The listing builds one solid part. Answer for the finished solid, in the listing's coordinates (mm). A direction names the side the tool comes from. Round coordinates to 2 decimals unless told otherwise and drop trailing zeros. Loops run counter-clockwise (first coordinate to the right, second up) from the corner with the lowest first, then second, coordinate; pieces in that order, holes last. Notation, with made-up numbers: M -26,-21 L 27,-21 A9 cw 27,-7 Z; hole C 83.5,-31 d6. An arc over 180 degrees is marked long. Answer as a JSON object with one key per item and string values.
Solid Edge part; units mm, degrees
sketch "Sketch1" plane through (0, 0, 0) normal (0, 0, 1) x (1, 0, 0)
  line L0 (-49.9158, -24.6721) -> (49.9158, -24.6721)
  line L1 (49.9158, -24.6721) -> (49.9158, 24.6721)
  line L2 (49.9158, 24.6721) -> (-49.9158, 24.6721)
  line L3 (-49.9158, 24.6721) -> (-49.9158, -24.6721)
extrude "Protrusion1" add sketch "Sketch1" along normal blind 31.771
draft "Draft_1" angle 4 neutral plane through (0, 0, 0) normal (0, 0, 1) pull direction (0, 0, 1) face at (49.9158, -16.9415, 26.1581) face at (34.2755, 24.6721, 26.1581) face at (-49.9158, 16.9415, 26.1581) face at (-34.2755, -24.6721, 26.1581)
fillet "Round_1" radius 6 8 edges at (-48.8049, -23.5613, 15.8855) (0, -22.4505, 31.771) (-47.6941, 0, 31.771) (-48.8049, 23.5613, 15.8855) (0, 22.4505, 31.771) (47.6941, 0, 31.771) (48.8049, -23.5613, 15.8855) (48.8049, 23.5613, 15.8855)
sketch "Sketch2" plane through (0, 0, 31.771) normal (0, 0, 1) x (0, 1, 0)
  circle A0 centre (11.4247, -36.4932) radius 4
extrude "ExtrudedCutout_1" cut sketch "Sketch2" against normal blind 65.3593
sketch "Sketch3" plane through (20.8309, 11.4247, 31.771) normal (0, 0, 1) x (-1, 0, 0)
  circle A0 centre (0, 0) radius 4
  circle A1 centre (15.6623, 0) radius 4
  circle A2 centre (31.3245, 0) radius 4
extrude "ExtrudedCutout_2" cut sketch "Sketch3" against normal blind 66.2854
sketch "Sketch4" plane through (0, 0, 31.771) normal (0, 0, 1) x (0, 1, 0)
  line L0 (-6.6575, 36.4932) -> (-6.6575, 18.7397)
  line L1 (-6.6575, 18.7397) -> (-14.5479, 18.7397)
  line L2 (-14.5479, 18.7397) -> (-14.5479, 36.4932)
  line L3 (-14.5479, 36.4932) -> (-6.6575, 36.4932)
extrude "ExtrudedCutout_3" cut sketch "Sketch4" against normal blind 15.8022
shell "Thin_Wall_1" thickness 1 removed faces 1 at (-34.2755, -15.9546, 0)
Item 1: The part is cut by section D-D (x = 23). Give the vertices of the cut face in (y, z).
Values follow:
{"outline": "M -24.67,0 L -23.67,0 L -21.84,26.12 A5 cw -16.86,30.77 L 6.92,30.77 L 6.92,0 L 8.06,0 L 8.06,31.77 L -16.86,31.77 A6 ccw -22.84,26.19 Z; M 14.79,0 L 15.93,0 L 15.93,30.77 L 16.86,30.77 A5 cw 21.84,26.12 L 23.67,0 L 24.67,0 L 22.84,26.19 A6 ccw 16.86,31.77 L 14.79,31.77 Z"}
Item 2: Determine the mould class of faces 3 (the face through (-0.62, -23.77, 12.91)), 4 (the face through (34, 15, 0)), 5 (the face through (-27, -15.548, 23)) for opening direction Y: released by +Y, released by -Y, zero draft, split by the parting line, or undercut.
Values follow:
{"face 3": "released by -Y", "face 4": "zero draft", "face 5": "undercut"}
Item 3: Which of the six approach directions +Z, -Z, +X, -X, +Y, -Y give full straight-line access (tool end or side, diameter ignored) to faces 1 (the face through (41.374, 10.341, 15.601)), 2 (the face through (5.69, 7.46, 16.11))?
Values follow:
{"face 1": "-Z", "face 2": "+Z, -Z"}
Item 4: The part is cut by section B-B (x = -25.5). Give the vertices of the cut face in (y, z), then the cut area to 3 significant figures.
Values follow:
{"outline": "M -24.67,0 L -23.67,0 L -21.84,26.12 A5 cw -16.86,30.77 L -15.55,30.77 L -15.55,14.97 L -5.66,14.97 L -5.66,30.77 L 16.86,30.77 A5 cw 21.84,26.12 L 23.67,0 L 24.67,0 L 22.84,26.19 A6 ccw 16.86,31.77 L -6.66,31.77 L -6.66,15.97 L -14.55,15.97 L -14.55,31.77 L -16.86,31.77 A6 ccw -22.84,26.19 Z", "area": "134 mm^2"}
Item 5: Straight lines are drawn through the part: line 1 (X direction, y = 16, z = 27); line 2 (Y direction, x = 34.5, z = 18); line 3 (Y direction, x = -9.5, z = 3). For each, find the intervals that lie inside material, in ascending order.
Values follow:
{"line 1": "-47.97 to -46.95, -12.51 to -8.48, 3.15 to 7.19, 18.81 to 22.85, 34.48 to 38.51, 46.95 to 47.97", "line 2": "-23.41 to -22.41, 6.84 to 7.96, 14.89 to 16.01, 22.41 to 23.41", "line 3": "-24.46 to -23.46, 6.52 to 7.55, 15.3 to 16.32, 23.46 to 24.46"}
Item 6: The part is cut by section A-A (y = -4). Give the vertices of the cut face in (x, z), then the cut area to 3 significant figures.
Values follow:
{"outline": "M -49.92,0 L -48.91,0 L -47.09,26.12 A5 cw -42.1,30.77 L 42.1,30.77 A5 cw 47.09,26.12 L 48.91,0 L 49.92,0 L 48.08,26.19 A6 ccw 42.1,31.77 L -42.1,31.77 A6 ccw -48.08,26.19 Z", "area": "153 mm^2"}
Item 7: The part is cut by section C-C (z = 12). Give the number of separate pieces and of enclosed holes in the cut face, then the cut area to 3 significant figures.
Values follow:
{"separate pieces": "5", "enclosed holes": "5", "area": "392 mm^2"}
Item 8: Flat-ended cylindrical pins translate along their axes: P1, Ø2, axis at y = -14, z = 22.5, coming from the +X side; P2, Ø2, axis at x = -11.5, y = -15, coming from the -Z side; P3, Ø1, axis at x = 39, z = 10, coming from the +Y side; P4, Ø7, axis at x = 5.17, y = 11.42, coming from the +Z side. Find the tip coordinate at first contact, or state that the pin passes through.
Values follow:
{"P1": "x = 48.41", "P2": "z = 30.77", "P3": "y = 24.01", "P4": "through"}
